Geometry: final body of the model. Coordinates: model frame, mm. A direction names the side the tool comes from. Coordinates: 2 decimals unless noted, no trailing zeros. Write each loop counter-clockwise with the first axis right and the second up, starting at its lowest first coordinate (ties: lowest second). Pieces come first, ordered by that corner, then holes. Notation, with made-up numbers: M 5,15 L 46,15 A24 cw 46,43 Z; hole C 5.5,-28.5 d4. An arc over 180 degrees is marked long. Write item = value, one per line. Start each with the question number.
Item 1: Pull-direction query (X, two-part tool) for faces 4 (the flat face through (100, -161, -49)), 5 (the flat face through (96, -336, -4)), 6 (the flat face through (8.5, -332, -4)); classes: +X half, -X half, draft (parallel to the pull), parting line (faces both ways), or undercut.
Item 2: First-contact query: pin 1 Ø6 at (y, z) = (-240, -37) entering from -X; pin 2 Ø1.9 at (x, z) = (71.5, -33) entering from +Y; pin 3 Ø1.4 at (x, z) = (71, -33) entering from -Y. Flat tips, straight axial feed; report the tip coordinate or a pass-through.
Item 3: Section B-B on x = 39.5. Output: boundary loops of the cut face in (y, z).
Item 4: Reachability of faces 1 (the flat face through (8.5, 4, -4)), 2 (the flat face through (4, 4, -8.5)), 3 (the flat face through (91.5, -332, -96)) from +Z, -Z, +X, -X, +Y, -Y: full face, straight path, thin tool, end or side. Return the list, or none.
Item 5: Section A-A on z = -69.5. Output: boundary loops of the cut face in (x, y), plus the area to 4 significant figures.
Item 6: Ray query, L1, parallel to Z at x = 71, y = -7; L2, parallel to Z at x = 29, y = -6; L3, parallel to Y at x = 80, z = -48.5. Return the intervals inside material, ascending. Write a range as [from, to].
from build123d import *

# Parameters (mm, degrees)
BOSS_EXTRUDE1_DEPTH      = 327.5
SKETCH30_R               = 1.2
CUT_EXTRUDE4_DEPTH       = 10
SKETCH31_W               = 8.5
SKETCH31_H               = 8.5
BOSS_EXTRUDE2_DEPTH      = 8.5
BOSS_EXTRUDE2_DEPTH_BACK = 336


with BuildPart() as part:
    # Sketch1 → Boss-Extrude1 (new body)
    with BuildSketch(Plane(origin=(0, 0, 0), x_dir=(1, 0, 0), z_dir=(0, 1, 0))):
        Polygon((0, 17), (0, 0), (17, 0), (83, 0), (100, 0), (100, 17), (100, 83), (100, 100), (83, 100), (17, 100), (0, 100), (0, 83), align=None)
    extrude(amount=-BOSS_EXTRUDE1_DEPTH)

    # Sketch30 → Cut-Extrude4 (cut)
    with BuildSketch(Plane(origin=(0, 0, 0), x_dir=(-1, 0, 0), z_dir=(0, 1, 0))):
        with Locations((-71, -50)):
            Circle(SKETCH30_R)
        with Locations((-29, -50)):
            Circle(SKETCH30_R)
        with Locations((-62, -33)):
            Circle(SKETCH30_R)
        with Locations((-71, -33)):
            Circle(SKETCH30_R)
    extrude(amount=-CUT_EXTRUDE4_DEPTH, mode=Mode.SUBTRACT)

    # Sketch31 → Boss-Extrude2 (add, two sides)
    with BuildSketch(Plane(origin=(0, -327.5, 0), x_dir=(-1, 0, 0), z_dir=(0, -1, 0))) as boss_extrude2_sk:
        with Locations((-4.25, 95.75)):
            Rectangle(SKETCH31_W, SKETCH31_H)
        with Locations((-95.75, 95.75)):
            Rectangle(SKETCH31_W, SKETCH31_H)
        with Locations((-4.25, 4.25)):
            Rectangle(SKETCH31_W, SKETCH31_H)
        with Locations((-95.75, 4.25)):
            Rectangle(SKETCH31_W, SKETCH31_H)
    extrude(amount=BOSS_EXTRUDE2_DEPTH)
    extrude(boss_extrude2_sk.sketch, amount=-BOSS_EXTRUDE2_DEPTH_BACK)


solid = part.part
Responses:
q1.face_4 = +X half
q1.face_5 = draft
q1.face_6 = undercut
q2.pin_1 = 0
q2.pin_2 = 0
q2.pin_3 = -327.5
q3.outline = M -327.5,-100 L 0,-100 L 0,0 L -327.5,0 Z
q4.face_1 = +Z, -Z, +Y
q4.face_2 = +X, -X, +Y
q4.face_3 = +Z, -Z, -Y
q5.outline = M 0,-327.5 L 100,-327.5 L 100,0 L 0,0 Z
q5.area = 32,750 mm²
q6.L1 = [-100, -51.2], [-48.8, -34.2], [-31.8, 0]
q6.L2 = [-100, -51.2], [-48.8, 0]
q6.L3 = [-327.5, 0]
